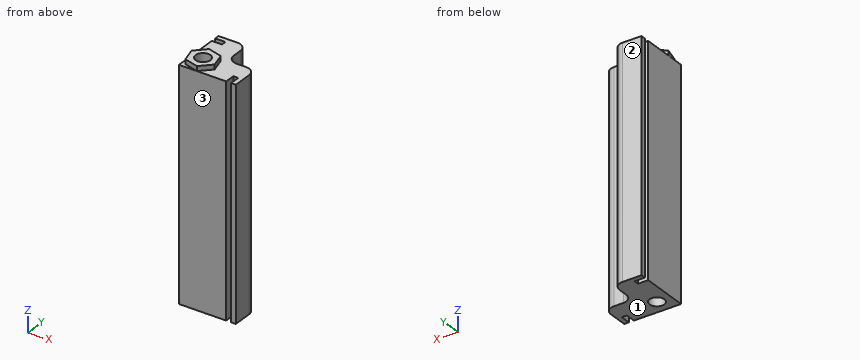
```python
from build123d import *

# Parameters (mm, degrees)
BOSS_EXTRUDE1_DEPTH = 152.4
SKETCH2_W           = 6.858
SKETCH2_H           = 3.302
SKETCH2_W_2         = 3.302
SKETCH2_H_2         = 6.858
CUT_EXTRUDE1_DEPTH  = 153.4
BOSS_EXTRUDE2_DEPTH = 3.175
FILLET1_R           = 6.35
SKETCH4_R           = 4.953
CUT_EXTRUDE2_DEPTH  = 156.575


with BuildPart() as part:
    # Sketch1 → Boss-Extrude1 (new body)
    with BuildSketch(Plane.XY):
        Polygon((0, 0), (0, 38.1), (19.05, 38.1), (19.05, 19.05), (38.1, 19.05), (38.1, 0), align=None)
    extrude(amount=BOSS_EXTRUDE1_DEPTH)

    # Sketch2 → Cut-Extrude1 (cut, through all)
    with BuildSketch(Plane.XY.offset(152.4)):
        with Locations((3.429, 33.274)):
            Rectangle(SKETCH2_W, SKETCH2_H)
        with Locations((33.274, 3.429)):
            Rectangle(SKETCH2_W_2, SKETCH2_H_2)
    extrude(amount=-CUT_EXTRUDE1_DEPTH, mode=Mode.SUBTRACT)

    # Sketch3 → Boss-Extrude2 (add)
    with BuildSketch(Plane.XY.offset(152.4)):
        Polygon((16.497783942, 16.497783942), (6.972783942, 19.05), (0, 12.077216058), (2.552216058, 2.552216058), (12.077216058, 0), (19.05, 6.972783942), align=None)
    extrude(amount=BOSS_EXTRUDE2_DEPTH)

    # Fillet1
    fillet1_edges = [part.edges().sort_by_distance(p)[0] for p in [
        (19.05, 38.1, 76.2),
        (19.05, 19.05, 76.2),
        (38.1, 19.05, 76.2),
    ]]
    fillet(fillet1_edges, radius=FILLET1_R)

    # Sketch4 → Cut-Extrude2 (cut, through all)
    with BuildSketch(Plane.XY.offset(155.575)):
        with Locations((9.525, 9.525)):
            Circle(SKETCH4_R)
    extrude(amount=-CUT_EXTRUDE2_DEPTH, mode=Mode.SUBTRACT)


solid = part.part
```
Read the model definition and answer for the solid it produces. Units are mm, in the model's axes. Face numbers are marked on the shaded views. Give positions to 0.01 mm unless a question says otherwise; leave off trailing zeros. Write each loop counter-clockwise with the first axis right and the second up, starting at its lowest first coordinate (ties: lowest second). Pieces come first, ordered by that corner, then holes. Notation, with made-up numbers: (19.5, 5.25) -> (67.5, 5.25) arc R17 ccw to (67.5, 18.25) -> close; hole circle Ø8 at (63, 62). An arc over 180 degrees is marked (long way). Answer as a JSON object with one key per item and string values.
1) For a pull along Y with two mould halves and no side action, classify the marked faces 1, 2 and 3 as pulls with the +Y half, pulls with the -Y half, needs draft (parallel to the pull), parting line crosses it, or undercut.
Findings below:
{"face 1": "needs draft", "face 2": "pulls with the +Y half", "face 3": "pulls with the -Y half"}
2) Section A-A on z = 17 is taken. Write down the section's boundary in (x, y) (3 decimals).
Findings below:
{"outline": "(0, 0) -> (31.623, 0) -> (31.623, 6.858) -> (34.925, 6.858) -> (34.925, 0) -> (38.1, 0) -> (38.1, 12.7) arc R6.35 ccw to (31.75, 19.05) -> (25.4, 19.05) arc R6.35 cw to (19.05, 25.4) -> (19.05, 31.75) arc R6.35 ccw to (12.7, 38.1) -> (0, 38.1) -> (0, 34.925) -> (6.858, 34.925) -> (6.858, 31.623) -> (0, 31.623) -> close; hole circle Ø9.906 at (9.525, 9.525)"}
3) Section C-C on y = 22.5 is taken. Write down the section's boundary in (x, z).
Findings below:
{"outline": "(0, 0) -> (19.75, 0) -> (19.75, 152.4) -> (0, 152.4) -> close"}
4) Flat-ended cylindrical pins translate along their axes: pin 1 Ø5 at (y, z) = (28, 38) entering from +X; pin 2 Ø1 at (y, z) = (33, 106) entering from -X; pin 3 Ø4 at (x, y) = (24, 20.5) entering from +Z. Find the tip coordinate at first contact, or state that the pin passes through.
Findings below:
{"pin 1": "stops at x = 19.05", "pin 2": "stops at x = 6.86", "pin 3": "stops at z = 152.4"}
5) Section B-B on y = 30 is taken. Write down the section's boundary in (x, z).
Findings below:
{"outline": "(0, 0) -> (19.05, 0) -> (19.05, 152.4) -> (0, 152.4) -> close"}
6) Straight lines are drawn through the part: probe 1 along Y at (x, z) = (4, 105.5) (3 decimals); probe 2 along Y at (x, z) = (10, 113). For each, find the intervals that lie inside material, in ascending order. Write a range as from..to.
Findings below:
{"probe 1": "y = 0..31.623, 34.925..38.1", "probe 2": "y = 0..4.59, 14.46..38.1"}
